```python
from build123d import *

# Parameters (mm, degrees)
SKETCH1_W                      = 25.4
SKETCH1_H                      = 25.4
SKETCH1_W_2                    = 20.828
SKETCH1_H_2                    = 20.828
BOSS_EXTRUDE1_DEPTH            = 285.75
F_3_16_0_1875_DIAMETER_HOLE7_D = 4.7625
F_0_257_DIAMETER_HOLE1_D       = 6.5278


with BuildPart() as part:
    # Sketch1 → Boss-Extrude1 (new body)
    with BuildSketch(Plane.XY):
        Rectangle(SKETCH1_W, SKETCH1_H)
        Rectangle(SKETCH1_W_2, SKETCH1_H_2, mode=Mode.SUBTRACT)
    extrude(amount=BOSS_EXTRUDE1_DEPTH)

    # 3/16 (0.1875) Diameter Hole7 (through all)
    with Locations(Plane(origin=(0, 12.7, 0), x_dir=(1, 0, 0), z_dir=(0, 1, 0))):
        with Locations((0, -273.05), (0, -247.65), (0, -12.7), (0, -38.1)):
            Hole(F_3_16_0_1875_DIAMETER_HOLE7_D / 2)

    # F (0.257) Diameter Hole1 (through all)
    with Locations(Plane(origin=(12.7, 0, 0), x_dir=(0, 0, -1), z_dir=(1, 0, 0))):
        with Locations((-180.975, 0), (-104.775, 0)):
            Hole(F_0_257_DIAMETER_HOLE1_D / 2)


solid = part.part
```
Can you work these out from the model? Positions are in its coordinate system, mm. A direction names the side the tool comes from. Give positions to 0.01 mm unless a question says otherwise; leave off trailing zeros. Loops run counter-clockwise (first coordinate to the right, second up) from the corner with the lowest first, then second, coordinate; pieces in that order, holes last. Notation, with made-up numbers: M 74.5,-4.5 L 94.5,-4.5 A17 ccw 94.5,10.5 Z; hole C 24.5,29 d4. An arc over 180 degrees is marked long. Answer in a Markdown table with one row per item.
1. Suppose I cut it at B-B on x = -8. Write out the boundary of the cut face in (y, z), plus the area to 3 significant figures.
Taken from the geometry:
| item | result |
|---|---|
| outline | M -12.7,0 L -10.41,0 L -10.41,285.75 L -12.7,285.75 Z; M 10.41,0 L 12.7,0 L 12.7,285.75 L 10.41,285.75 Z |
| area | 1,310 mm² |
2. Suppose I cut it at D-D on z = 247.65. Write out the boundary of the cut face in (x, y).
Taken from the geometry:
| item | result |
|---|---|
| outline | M -12.7,-12.7 L -2.38,-12.7 L -2.38,-10.41 L -10.41,-10.41 L -10.41,10.41 L -2.38,10.41 L -2.38,12.7 L -12.7,12.7 Z; M 2.38,-12.7 L 12.7,-12.7 L 12.7,12.7 L 2.38,12.7 L 2.38,10.41 L 10.41,10.41 L 10.41,-10.41 L 2.38,-10.41 Z |
3. Suppose I cut it at C-C on z = 156. Write out the boundary of the cut face in (x, y), plus the area to 3 significant figures.
Taken from the geometry:
| item | result |
|---|---|
| outline | M -12.7,-12.7 L 12.7,-12.7 L 12.7,12.7 L -12.7,12.7 Z; hole M -10.41,-10.41 L 10.41,-10.41 L 10.41,10.41 L -10.41,10.41 Z |
| area | 211 mm² |
4. If I drill on line 1 along Z through (x, y) = (0, -11.85); line 2 along Y through (x, z) = (5.75, 95), over which ranges is the centre line in solid material (lowest first)?
Taken from the geometry:
| item | result |
|---|---|
| line 1 | z = 0 to 10.32, 15.08 to 35.72, 40.48 to 245.27, 250.03 to 270.67, 275.43 to 285.75 |
| line 2 | y = -12.7 to -10.41, 10.41 to 12.7 |
5. Suppose I cut it at A-A on y = 0. Write out the boundary of the cut face in (x, z), plus the area to 3 significant figures.
Taken from the geometry:
| item | result |
|---|---|
| outline | M -12.7,0 L -10.41,0 L -10.41,101.51 L -12.7,101.51 Z; M -12.7,108.04 L -10.41,108.04 L -10.41,177.71 L -12.7,177.71 Z; M -12.7,184.24 L -10.41,184.24 L -10.41,285.75 L -12.7,285.75 Z; M 10.41,0 L 12.7,0 L 12.7,101.51 L 10.41,101.51 Z; M 10.41,108.04 L 12.7,108.04 L 12.7,177.71 L 10.41,177.71 Z; M 10.41,184.24 L 12.7,184.24 L 12.7,285.75 L 10.41,285.75 Z |
| area | 1,250 mm² |
6. Thinking about a two-plate mould opening in X: for faces 3 (the flat face through (0, -12.7, 141)), 4 (the flat face through (-12.7, 0, 141)), 5 (the cylindrical face through (0.31, 11.54, 10.34)), which applies, released by +X, released by -X, zero draft, split by the parting line, or undercut?
Taken from the geometry:
| item | result |
|---|---|
| face 3 | zero draft |
| face 4 | released by -X |
| face 5 | undercut |
7. Which directions (+Z, -Z, +X, -X, +Y, -Y) give clear straight access to the entire face, cutting with the end or side of a thin tool? Please do faces 1 (the cylindrical face through (-11.573, 0.144, 101.514)), 2 (the flat face through (0, 10.414, 141)).
Taken from the geometry:
| item | result |
|---|---|
| face 1 | +X, -X |
| face 2 | +Z, -Z |
